```python
from build123d import *

# Parameters (mm, degrees)
SKETCH1_W           = 13
SKETCH1_H           = 40
BOSS_EXTRUDE1_DEPTH = 5
SKETCH2_R           = 2.5
BOSS_EXTRUDE2_DEPTH = 9
LPATTERN1_COUNT     = 2
LPATTERN1_PITCH     = 20


with BuildPart() as part:
    # Sketch1 → Boss-Extrude1 (new body)
    with BuildSketch(Plane(origin=(0, 0, 0), x_dir=(0, 1, 0), z_dir=(0, 0, 1))):
        Rectangle(SKETCH1_W, SKETCH1_H)
    extrude(amount=BOSS_EXTRUDE1_DEPTH)


with BuildPart() as body_2:
    # Sketch2 → Boss-Extrude2 (new body)
    with BuildSketch(Plane.YZ.offset(20)):
        with BuildLine():
            Line((-6.5, 0), (-9.5, 0))
            ThreePointArc((-9.5, 0), (-12.328427125, 1.171572875), (-13.5, 4))
            Line((-13.5, 4), (-13.5, 7.272429229))
            ThreePointArc((-13.5, 7.272429229), (-13.475070012, 7.494326663), (-13.401523057, 7.705160297))
            Line((-13.401523057, 7.705160297), (-12.572289088, 9.432731068))
            ThreePointArc((-12.572289088, 9.432731068), (-12.203339467, 9.846383798), (-11.67076603, 10))
            Line((-11.67076603, 10), (-8.32923397, 10))
            ThreePointArc((-8.32923397, 10), (-7.796660533, 9.846383798), (-7.427710912, 9.432731068))
            Line((-7.427710912, 9.432731068), (-6.598476943, 7.705160297))
            ThreePointArc((-6.598476943, 7.705160297), (-6.524929988, 7.494326663), (-6.5, 7.272429229))
            Line((-6.5, 7.272429229), (-6.5, 5))
            Line((-6.5, 5), (-6.5, 0))
        make_face()
        with Locations(Location((-10, 6, 0), (0, 0, 270))):
            Circle(SKETCH2_R, mode=Mode.SUBTRACT)
    boss_extrude2 = extrude(amount=-BOSS_EXTRUDE2_DEPTH)


with BuildPart() as lpattern1_1:
    # LPattern1: Boss-Extrude2 ×2
    with Locations(*[(-i * LPATTERN1_PITCH, 0, 0) for i in range(1, LPATTERN1_COUNT)]):
        add(boss_extrude2)


with BuildPart() as body_2_1:
    add(body_2.part)

    # Combine1: union LPattern1_1, part
    add(lpattern1_1.part)
    add(part.part)


solid = body_2_1.part
```
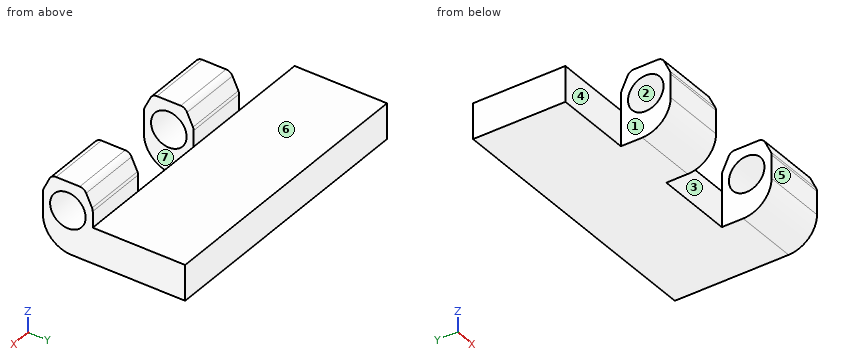
Here's how the part is built. I have some questions about the finished solid (model axes, mm). Face numbers are marked on the shaded views. A direction names the side the tool comes from. Round coordinates to 2 decimals unless told otherwise and drop trailing zeros. Write each loop counter-clockwise with the first axis right and the second up, starting at its lowest first coordinate (ties: lowest second). Pieces come first, ordered by that corner, then holes.
Q1. If we section it at B-B on x = 16.5: Write out the boundary of the cut face in (y, z).
Q2. Please list where these lines run through material, in increasing order: probe 1 along Y at (x, z) = (15.25, 6); probe 2 along Y at (x, z) = (-14.5, 4.25); probe 3 along Z at (x, y) = (-10.5, -5.25).
Q3. If we section it at D-D on z = 6: Write out the boundary of the cut face in (x, y), plus the area to 3 significant figures.
Q4. If we section it at A-A on z = 9: Write out the boundary of the cut face in (x, y).
Q5. Which directions (+Z, -Z, +X, -X, +Y, -Y) give clear straight access to the entire face, cutting with the end or side of a thin tool? Please do the marked faces 4, 5, 6 and 7.
Q6. Will these pins go through, and if not, where does the flat tip stop? P1, Ø5.5, axis at x = -15, z = 2.5, coming from the -Y side; P2, Ø5.5, axis at y = -10, z = 7.5, coming from the -X side; P3, Ø2.5, axis at x = 16, z = 6.5, coming from the +Y side.
Q7. If we mould it in two halves opening along X, with no side actions, what happens to the marked faces 1, 2 and 3? For each: +X half, -X half, draft (parallel to the pull), parting line (faces both ways), or undercut.
Q8. If we section it at C-C on y = -10: Write out the boundary of the cut face in (x, z), plus the area to 3 significant figures.
Answer below:
1. outline: (-13.5, 4) arc R4 ccw to (-9.5, 0) - (6.5, 0) - (6.5, 5) - (-6.5, 5) - (-6.5, 7.27) arc R1 ccw to (-6.6, 7.71) - (-7.43, 9.43) arc R1 ccw to (-8.33, 10) - (-11.67, 10) arc R1 ccw to (-12.57, 9.43) - (-13.4, 7.71) arc R1 ccw to (-13.5, 7.27) - close; hole circle Ø5 at (-10, 6)
2. probe 1: y = -13.5 to -12.5, -7.5 to -6.5
2. probe 2: y = -6.5 to 6.5
2. probe 3: z = 0 to 5
3. outline: (-9, -13.5) - (0, -13.5) - (0, -12.5) - (-9, -12.5) - close; (-9, -7.5) - (0, -7.5) - (0, -6.5) - (-9, -6.5) - close; (11, -13.5) - (20, -13.5) - (20, -12.5) - (11, -12.5) - close; (11, -7.5) - (20, -7.5) - (20, -6.5) - (11, -6.5) - close
3. area: 36.0 mm2
4. outline: (-9, -12.78) - (0, -12.78) - (0, -7.22) - (-9, -7.22) - close; (11, -12.78) - (20, -12.78) - (20, -7.22) - (11, -7.22) - close
5. face 4: +Z, -Z, -X, -Y
5. face 5: +Z, -Z, +X, -X, -Y
5. face 6: +Z, +X, -X, +Y
5. face 7: +Z, -Z, -Y
6. P1: stops at y = -6.5
6. P2: stops at x = -9
6. P3: stops at y = -6.5
7. face 1: -X half
7. face 2: draft
7. face 3: undercut
8. outline: (-9, 0.03) - (0, 0.03) - (0, 3.5) - (-9, 3.5) - close; (-9, 8.5) - (0, 8.5) - (0, 10) - (-9, 10) - close; (11, 0.03) - (20, 0.03) - (20, 3.5) - (11, 3.5) - close; (11, 8.5) - (20, 8.5) - (20, 10) - (11, 10) - close
8. area: 89.4 mm2
